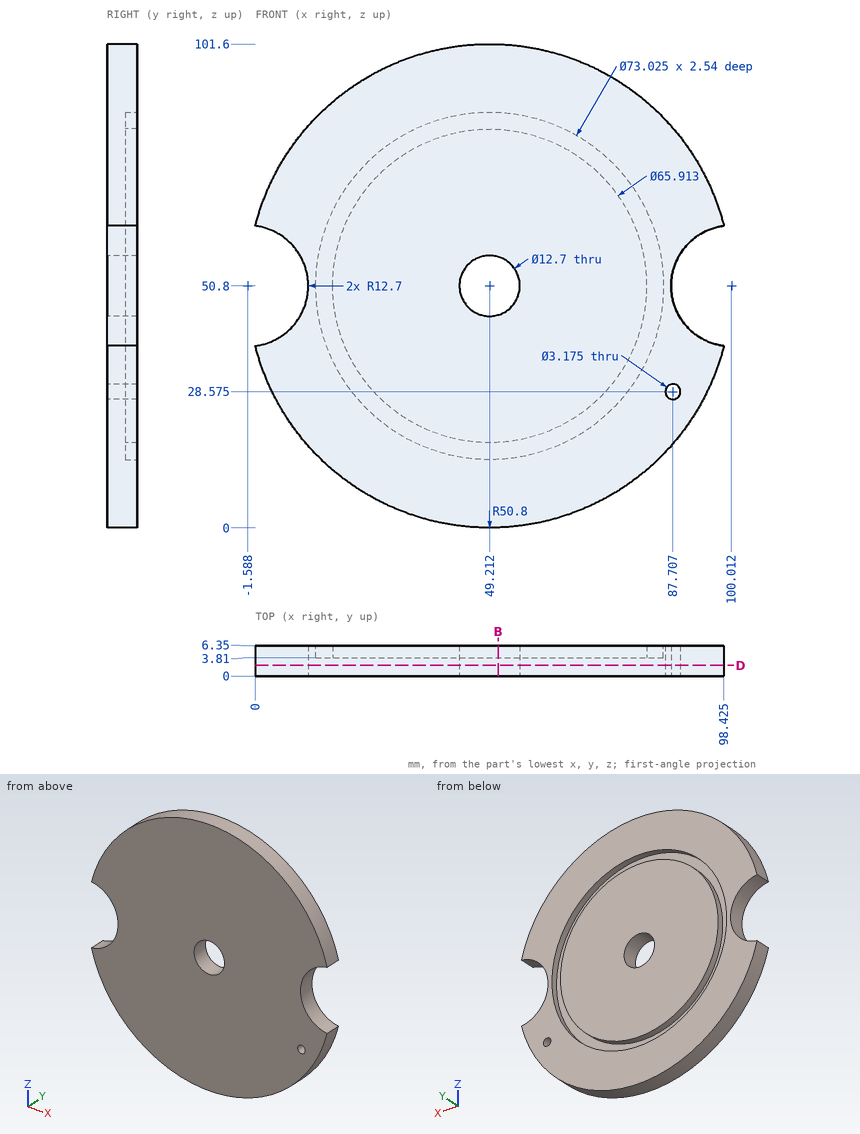
Input: dimensioned drawing with shaded views. Units: mm. Origin: part minimum x, y, z. Give positions to 0.01 mm unless a question says otherwise; leave off trailing zeros. Loops run counter-clockwise (first coordinate to the right, second up) from the corner with the lowest first, then second, coordinate; pieces in that order, holes last. Notation, with made-up numbers: (8.5, -9.75) -> (39.5, -9.75) arc R18 ccw to (39.5, 0.25) -> close; hole circle Ø11 at (70.25, -28). An arc over 180 degrees is marked (long way). Return JSON: item names as keys, results as strings.
Item 1: Section D-D, the plane y = 2.25. Count the separate pieces of the cut face and the enclosed holes in it, plus the area to 3 significant figures.
Filled in:
{"separate pieces": "1", "enclosed holes": "2", "area": "7,490 mm^2"}
Item 2: Pin query (flat end, axial travel): P1, Ø7.5, axis at x = 49.21, z = 50.8, coming from the -Y side; P2, Ø3, axis at x = 33, y = 4, coming from the -Z side; P3, Ø1, axis at y = 1, z = 33.5, coming from the -X side; P4, Ø1, axis at y = 3.5, z = 40, coming from the -X side. Return the tip coordinate at first contact, or that it passes through.
Filled in:
{"P1": "through", "P2": "z = 2.18", "P3": "x = 1.27", "P4": "x = 4.21"}
Item 3: Section B-B, the plane x = 51. Output: boundary loops of the cut face in (y, z).
Filled in:
{"outline": "(0, 0.03) -> (6.35, 0.03) -> (6.35, 14.33) -> (3.81, 14.33) -> (3.81, 17.89) -> (6.35, 17.89) -> (6.35, 44.71) -> (0, 44.71) -> close; (0, 56.89) -> (6.35, 56.89) -> (6.35, 83.71) -> (3.81, 83.71) -> (3.81, 87.27) -> (6.35, 87.27) -> (6.35, 101.57) -> (0, 101.57) -> close"}
Item 4: Line query: line 1 (Z direction, x = 49.5, y = 5.5) (1 decimal); line 2 (Z direction, x = 32.5, y = 5.5) (1 decimal); line 3 (X direction, y = 5.5, z = 31) (1 decimal). Output: solid intervals per line, ascending.
Filled in:
{"line 1": "0 to 14.3, 17.8 to 44.5, 57.1 to 83.8, 87.3 to 101.6", "line 2": "2.8 to 18.3, 22.4 to 79.2, 83.3 to 98.8", "line 3": "2.4 to 18.5, 22.9 to 75.6, 79.9 to 96"}
